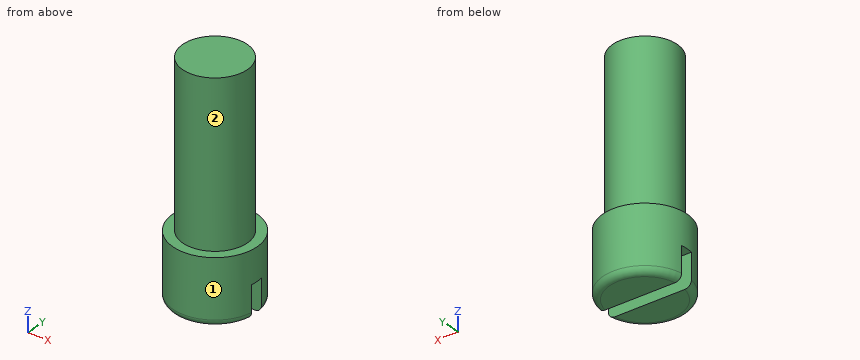
from build123d import *

# Parameters (mm, degrees)
F0_R     = 50
F1_DEPTH = 350
F0_R_2   = 65
F2_DEPTH = 100
F3_R     = 10
F4_W     = 20
F4_H     = 53.732174
F5_DEPTH = 150


with BuildPart() as f1:
    # F0 (on Top) → F1 (new body)
    with BuildSketch(Plane.XY):
        Circle(F0_R)
    extrude(amount=F1_DEPTH)

    # F0 (on Top) → F2 (join)
    with BuildSketch(Plane.XY):
        Circle(F0_R_2)
        Circle(F0_R, mode=Mode.SUBTRACT)
    extrude(amount=F2_DEPTH)

    # F3
    f3_edges = [f1.edges().sort_by_distance(p)[0] for p in [
        (-65, 0, 0),
    ]]
    fillet(f3_edges, radius=F3_R)

    # F4 (on Right) → F5 (cut, symmetric)
    with BuildSketch(Plane.YZ):
        with Locations((0, 23.133913)):
            Rectangle(F4_W, F4_H)
    extrude(amount=F5_DEPTH, both=True, mode=Mode.SUBTRACT)


solid = f1.part
Read the model definition and answer for the solid it produces. Units are mm, in the model's axes. Face numbers are marked on the shaded views. A direction names the side the tool comes from. Coordinates: 2 decimals unless noted, no trailing zeros. Order: outer loops, then holes, each group sorted by start corner. A loop starts at its lowest first (then second) coordinate and runs counter-clockwise, first axis right, second up. Notation, with made-up numbers: (16.25, -21.75) - (64.25, -21.75) arc R9 cw to (64.25, -6.75) - close; hole circle Ø3 at (79, 75.5). An arc over 180 degrees is marked (long way). Use one line per item in the form item = value.
(1) Section A-A, the plane y = 0 is taken. Give the vertices of the cut face in (x, z), then the cut area to 3 significant figures.
Computed values:
outline = (-65, 50) - (65, 50) - (65, 100) - (50, 100) - (50, 350) - (-50, 350) - (-50, 100) - (-65, 100) - close
area = 31,500 mm²
(2) Given pin 1 Ø10 at (x, z) = (-52, 92.5) entering from +Y; pin 2 Ø1.5 at (x, z) = (21.5, 56.5) entering from +Y; pin 3 Ø3 at (y, z) = (38, 239.5) entering from +X, each flat-ended and moving along its own axis, determine where each tip first touches the part or whether it passes through.
Computed values:
pin_1 = 44.9
pin_2 = 61.6
pin_3 = 34.17
(3) Which of the six approach directions +Z, -Z, +X, -X, +Y, -Y give full straight-line access (tool end or side, diameter ignored) to the marked faces 1 and 2?
Computed values:
face_1 = +Z, -Z
face_2 = +Z
(4) Section C-C, the plane z = 290 is taken. Give the vertices of the cut face in (x, y), then the cut area to 3 significant figures.
Computed values:
outline = circle Ø100 at (0, 0)
area = 7,850 mm²
(5) Straight lines are drawn through the part: L1, parallel to Z at x = -33, y = 0.5; L2, parallel to Z at x = -46, y = -24; L3, parallel to Y at x = -50.5, z = 45. For each, find the intervals that lie inside material, in ascending order.
Computed values:
L1 = 50 to 350
L2 = 0 to 100
L3 = -40.92 to -10, 10 to 40.92
(6) Section B-B, the plane x = 0 is taken. Give the vertices of the cut face in (y, z), then the cut area to 3 significant figures.
Computed values:
outline = (-65, 10) arc R10 ccw to (-55, 0) - (-10, 0) - (-10, 50) - (10, 50) - (10, 0) - (55, 0) arc R10 ccw to (65, 10) - (65, 100) - (50, 100) - (50, 350) - (-50, 350) - (-50, 100) - (-65, 100) - close
area = 37,000 mm²
